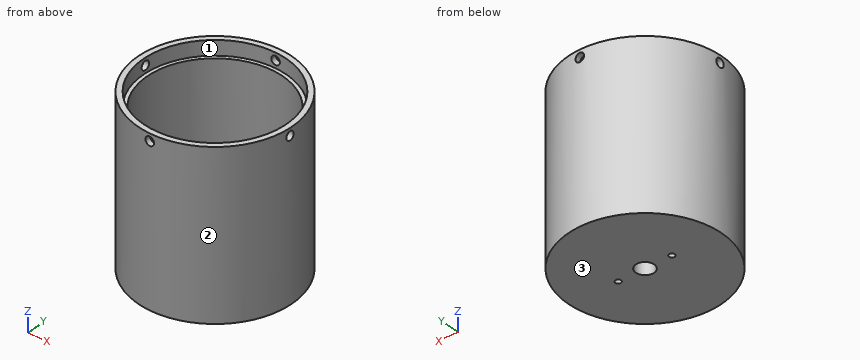
Autodesk Inventor part; units mm, degrees
ref_plane "Arbeitsebene1" through (0, -21, 0) normal (0, 1, 0) x (-1, 0, 0)
ref_plane "YZ Plane" through (0, 0, 0) normal (1, 0, 0) x (0, 1, 0)
ref_plane "XY Plane" through (0, 0, 0) normal (0, 0, 1) x (1, 0, 0)
sketch "Skizze1" plane through (0, 0, 0) normal (0, 0, 1) x (1, 0, 0)
  line L0 (-29.4, 0) -> (29.4, 0)
  line L1 (0, -29.4) -> (0, 29.4)
  circle A0 centre (0, 0) radius 21
  dimension "d0" = 42
extrude "Extrusion1" add sketch "Skizze1" along normal blind 5
sketch "Skizze2" plane through (0, 0, 5) normal (0, 0, 1) x (1, 0, 0)
  circle A0 centre (0, 0) radius 21
  circle A1 centre (0, 0) radius 21
  circle A2 centre (0, 0) radius 19.5
  dimension "d3" = 39
extrude "Extrusion2" add sketch "Skizze2" along normal blind 40
sketch "Skizze3" plane through (0, 0, 0) normal (0, 0, -1) x (-1, 0, 0)
  line L0 (29.4, 0) -> (-29.4, 0)
  line L1 (0, -29.4) -> (0, 29.4)
  point P0 (-7.5, 0)
  point P1 (7.5, 0)
  dimension "d6" = 15
hole "Bohrung1" at (7.5, 0, 0) at (-7.5, 0, 0) direction (0, 0, 1) diameter 1.567 end through all
hole "Bohrung2" at (0, 0, 0) direction (0, 0, 1) diameter 5 end through all
ref_plane "Arbeitsebene1" through (0, -21, 0) normal (0, 1, 0) x (-1, 0, 0)
sketch "Skizze4" plane through (0, -21, 0) normal (0, 1, 0) x (-1, 0, 0)
  line L0 (29.4, 0) -> (-29.4, 0)
  line L1 (0, -9) -> (0, 54)
  line L2 (21, 45) -> (-21, 45)
  point P0 (0, 0)
  point P1 (0, 43)
  dimension "d23" = 2
hole "Bohrung3" at (0, -21, 43) direction (0, 1, 0) diameter 2.4 end through all
pattern_circular "Runde Anordnung1" count 4 over 360 about axis through (0, 0, -10) along (0, 0, 1) of "Bohrung3"
sketch "Skizze5" plane through (0, 0, 5) normal (0, 0, 1) x (1, 0, 0)
  circle A0 centre (0, 0) radius 19.5
  circle A1 centre (0, 0) radius 18.5
  dimension "d34" = 37
extrude "Extrusion3" add sketch "Skizze5" along normal blind 36
properties part number "13_1087_060"
Work out the finished part from the listing and answer in its coordinate system (mm). Face numbers are marked on the shaded views. Coordinates: 2 decimals unless noted, no trailing zeros. Write each loop counter-clockwise with the first axis right and the second up, starting at its lowest first coordinate (ties: lowest second). Pieces come first, ordered by that corner, then holes.
Q1. A cutting plane is placed at A-A, the plane x = 0. Give the vertices of the cut face in (y, z).
Q2. A cutting plane is placed at C-C, the plane x = -7.5. Give the vertices of the cut face in (y, z).
Q3. Find the intervals of material crossed by line 1 (X direction, y = 0, z = 1); line 2 (X direction, y = -0.5, z = 23.5); line 3 (Z direction, x = -6, y = -3.5), in increasing order.
Q4. A cutting plane is placed at D-D, the plane z = 43. Give the vertices of the cut face in (x, y).
Q5. Each of these flat-tipped pins is pushed along its axis until it touches: pin 1 Ø3 at (y, z) = (14, 34) entering from -X; pin 2 Ø8 at (x, z) = (6.5, 36) entering from +Y; pin 3 Ø11 at (x, y) = (6, -5) entering from +Z. Where does it stop, or does it pass through?
Q6. Determine the mould class of the marked faces 1, 2 and 3 for opening direction Y: released by +Y, released by -Y, zero draft, split by the parting line, or undercut.
Q7. A cutting plane is placed at B-B, the plane y = 0. State how many separate pieces and enclosed holes the cut face has, then the cut area to 3 significant figures.
Findings below:
1. outline: (-21, 0) - (-2.5, 0) - (-2.5, 5) - (-18.5, 5) - (-18.5, 41) - (-19.5, 41) - (-19.5, 41.8) - (-21, 41.8) - close; (-21, 44.2) - (-19.5, 44.2) - (-19.5, 45) - (-21, 45) - close; (2.5, 0) - (21, 0) - (21, 41.8) - (19.5, 41.8) - (19.5, 41) - (18.5, 41) - (18.5, 5) - (2.5, 5) - close; (19.5, 44.2) - (21, 44.2) - (21, 45) - (19.5, 45) - close
2. outline: (-19.62, 0) - (-0.78, 0) - (-0.78, 5) - (-16.91, 5) - (-16.91, 41) - (-18, 41) - (-18, 45) - (-19.62, 45) - close; (0.78, 0) - (19.62, 0) - (19.62, 45) - (18, 45) - (18, 41) - (16.91, 41) - (16.91, 5) - (0.78, 5) - close
3. line 1: x = -21 to -8.28, -6.72 to -2.5, 2.5 to 6.72, 8.28 to 21
3. line 2: x = -20.99 to -18.49, 18.49 to 20.99
3. line 3: z = 0 to 5
4. outline: (-20.97, -1.2) arc R21 ccw to (-1.2, -20.97) - (-1.2, -19.46) arc R19.5 cw to (-19.46, -1.2) - close; (-20.97, 1.2) - (-19.46, 1.2) arc R19.5 cw to (-1.2, 19.46) - (-1.2, 20.97) arc R21 ccw to start; (1.2, -20.97) arc R21 ccw to (20.97, -1.2) - (19.46, -1.2) arc R19.5 cw to (1.2, -19.46) - close; (1.2, 19.46) arc R19.5 cw to (19.46, 1.2) - (20.97, 1.2) arc R21 ccw to (1.2, 20.97) - close
5. pin 1: stops at x = -16.87
5. pin 2: stops at y = 20.85
5. pin 3: stops at z = 5
6. face 1: undercut
6. face 2: split by the parting line
6. face 3: zero draft
7. separate pieces: 6
7. enclosed holes: 0
7. area: 354 mm2
